Verification items for this drawing (mm, ordinates from the low corner). A direction names the side the tool comes from. Round coordinates to 2 decimals unless told otherwise and drop trailing zeros. Loops run counter-clockwise (first coordinate to the right, second up) from the corner with the lowest first, then second, coordinate; pieces in that order, holes last. Notation, with made-up numbers: M -26.75,38 L -9.75,38 A23 cw -9.75,62 Z; hole C -29,61 d4. An arc over 180 degrees is marked long. One line per item, written item: value.
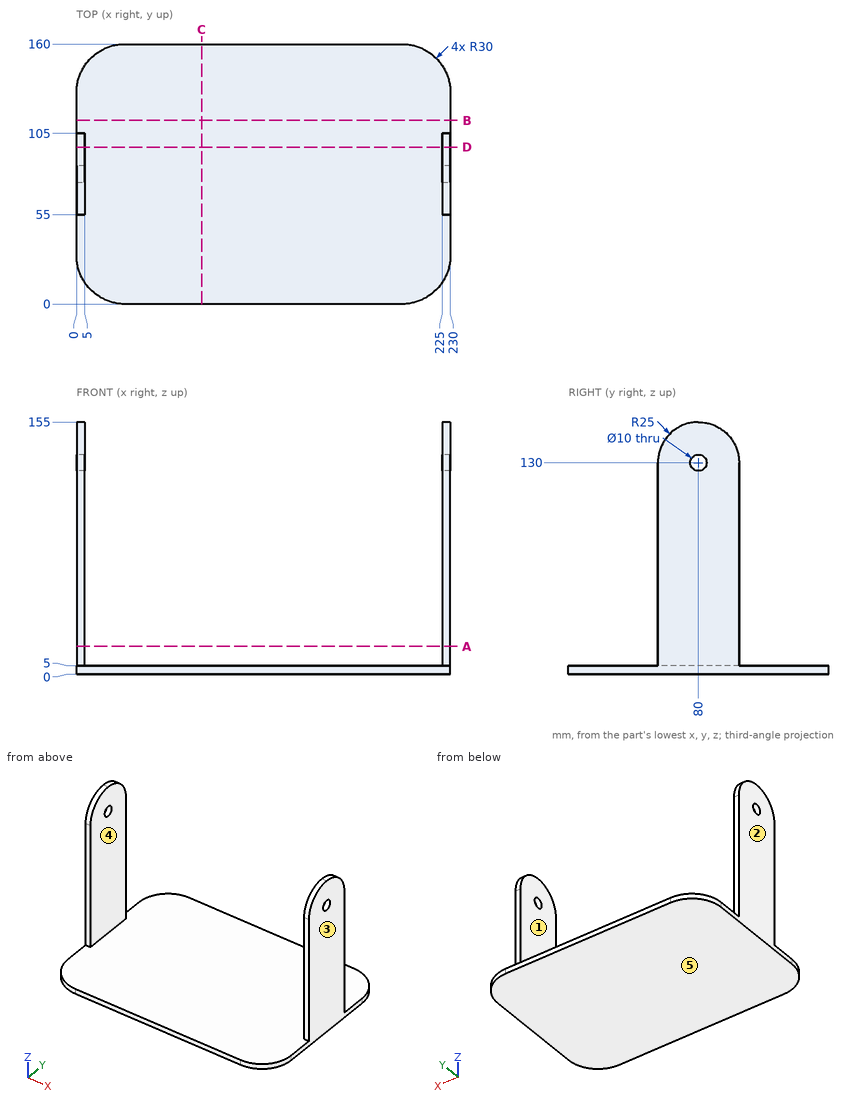
(1) Depth check by flat-ended pin: pin 1 Ø4 at (x, z) = (228, 38.5) entering from -Y; pin 2 Ø6 at (y, z) = (80, 130) entering from -X; pin 3 Ø8 at (x, y) = (137, 143) entering from +Z; pin 4 Ø5.5 at (x, z) = (1.5, 50.5) entering from +Y. Enter the tip coordinate at first touch or a pass-through.
Completed:
pin 1: stops at y = 55
pin 2: passes through
pin 3: stops at z = 5
pin 4: stops at y = 105
(2) Sectioned sample at D-D on y = 96.5. Enter the section's corners in (x, z), and give its area (3 significant figures).
Completed:
outline: M 0,0 L 230,0 L 230,148.78 L 225,148.78 L 225,5 L 5,5 L 5,148.78 L 0,148.78 Z
area: 2,590 mm^2
(3) Sectioned sample at B-B on y = 113. Enter the section's corners in (x, z).
Completed:
outline: M 0,0 L 230,0 L 230,5 L 0,5 Z
(4) Sectioned sample at A-A on z = 17. Enter the section's corners in (x, y).
Completed:
outline: M 0,55 L 5,55 L 5,105 L 0,105 Z; M 225,55 L 230,55 L 230,105 L 225,105 Z
(5) Tool access check on the marked faces 4 and 5. Record the directions out of +Z, -Z, +X, -X, +Y, -Y that give a thin tool (end or side, any length) a straight path to the whole face; none if there is none.
Completed:
face 4: +Z, +Y, -Y
face 5: -Z, +X, -X, +Y, -Y
(6) Thickness scan on L1, parallel to X at y = 92, z = 23.5; L2, parallel to Z at x = 34, y = 24.5. Record the ranges inside material, lowest first. Write a range as from..to.
Completed:
L1: x = 0..5, 225..230
L2: z = 0..5
(7) Mould release check, pull along X, two halves, no side actions. Record for the marked faces 1, 2 and 3: +X half, -X half, draft (parallel to the pull), parting line (faces both ways), or undercut.
Completed:
face 1: undercut
face 2: -X half
face 3: +X half
(8) Sectioned sample at C-C on x = 77. Enter the section's corners in (y, z), and give its area (3 significant figures).
Completed:
outline: M 0,0 L 160,0 L 160,5 L 0,5 Z
area: 800 mm^2
